Here's how the part is built. I have some questions about the finished solid (model axes, mm). Face numbers are marked on the shaded views. A direction names the side the tool comes from. Give positions to 0.01 mm unless a question says otherwise; leave off trailing zeros. Write each loop counter-clockwise with the first axis right and the second up, starting at its lowest first coordinate (ties: lowest second). Pieces come first, ordered by that corner, then holes. Notation, with made-up numbers: (58, 79) - (107, 79) arc R20 ccw to (107, 97) - close; hole circle Ø3 at (83, 87.5). An arc over 180 degrees is marked (long way). Use one line per item in the form item = value. Start each with the question number.
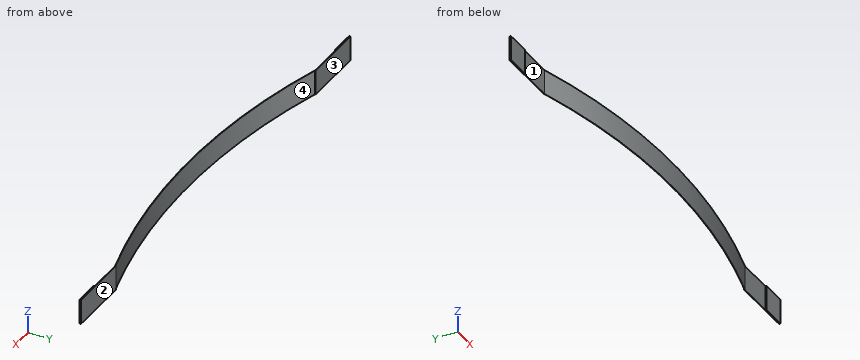
from build123d import *

# Parameters (mm, degrees)
SKETCH1_W           = 49.8
SKETCH1_H           = 1
BOSS_EXTRUDE1_DEPTH = 50.8


with BuildPart() as part:
    # Sketch1 → Boss-Extrude1 (new body)
    with BuildSketch(Plane.XY):
        with BuildLine():
            Line((-444.5, 1), (-495.3, 1))
            Line((-495.3, 1), (-495.3, -2))
            Line((-495.3, -2), (-444.5, -2))
            Line((-444.5, -2), (-443.5, -2))
            Line((-443.5, -2), (-443.5, 0))
            Line((-443.5, 0), (-368.3, 0))
            ThreePointArc((-368.3, 0), (0, -51.8), (368.3, 0))
            Line((368.3, 0), (443.5, 0))
            Line((443.5, 0), (443.5, -2))
            Line((443.5, -2), (444.5, -2))
            Line((444.5, -2), (495.3, -2))
            Line((495.3, -2), (495.3, 1))
            Line((495.3, 1), (444.5, 1))
            Line((444.5, 1), (368.3, 1))
            Line((368.3, 1), (367.3, 1))
            Line((367.3, 1), (367.3, 0))
            ThreePointArc((367.3, 0), (0, -50.8), (-367.3, 0))
            Line((-367.3, 0), (-367.3, 1))
            Line((-367.3, 1), (-368.3, 1))
            Line((-368.3, 1), (-444.5, 1))
        make_face()
        with Locations((-469.4, -0.5)):
            Rectangle(SKETCH1_W, SKETCH1_H, mode=Mode.SUBTRACT)
        with Locations((469.4, -0.5)):
            Rectangle(SKETCH1_W, SKETCH1_H, mode=Mode.SUBTRACT)
    extrude(amount=BOSS_EXTRUDE1_DEPTH)


solid = part.part
1. Please list where these lines run through material, in increasing order: line 1 (Y direction, x = -439, z = 35); line 2 (Y direction, x = -82, z = 48).
2. For the marked faces 1 and 2, which set-ups out of +Z, -Z, +X, -X, +Y, -Y let a thin tool reach every point of the face, with its end or its side?
3. I want a section at B-B, the plane y = -10. List the corners of the cut face in (x, z) for me.
4. I want a section at C-C, the plane x = 425.5. List the corners of the cut face in (y, z) for me.
5. We'd pull the mould along X, two halves only. Please class the marked faces 3 and 4: pulls with the +X half, pulls with the -X half, needs draft (parallel to the pull), parting line crosses it, or undercut.
6. For P1, Ø15, axis at x = 416.5, z = 27, coming from the -Y side; P2, Ø4, axis at x = 226, z = 21, coming from the +Y side; P3, Ø15, axis at x = 469, z = 22.5, coming from the -Y side, each with a flat end and sliding along its axis, tell me the tip position at first contact or that it passes through.
7. I want a section at A-A, the plane z = 17. List the corners of the cut face in (x, y) for me.
Result sheet:
q1.line_1 = 0 to 1
q1.line_2 = -49.28 to -48.31
q2.face_1 = +Z, -Z, -Y
q2.face_2 = +Z, -Z, +X, -X, +Y
q3.outline = (-331.48, 0) - (-329.79, 0) - (-329.79, 50.8) - (-331.48, 50.8) - close; (329.79, 0) - (331.48, 0) - (331.48, 50.8) - (329.79, 50.8) - close
q4.outline = (0, 0) - (1, 0) - (1, 50.8) - (0, 50.8) - close
q5.face_3 = needs draft
q5.face_4 = undercut
q6.P1 = 0
q6.P2 = -31.45
q6.P3 = -2
q7.outline = (-495.3, -2) - (-443.5, -2) - (-443.5, 0) - (-368.3, 0) arc R1335.21 ccw to (368.3, 0) - (443.5, 0) - (443.5, -2) - (495.3, -2) - (495.3, 1) - (367.3, 1) - (367.3, 0) arc R1353.25 cw to (-367.3, 0) - (-367.3, 1) - (-495.3, 1) - close; hole (-494.3, -1) - (-444.5, -1) - (-444.5, 0) - (-494.3, 0) - close; hole (444.5, -1) - (494.3, -1) - (494.3, 0) - (444.5, 0) - close
